Input: part model. Units: mm. Frame: model coordinates. A direction names the side the tool comes from. Coordinates: 2 decimals unless noted, no trailing zeros. Loops run counter-clockwise (first coordinate to the right, second up) from the corner with the lowest first, then second, coordinate; pieces in that order, holes last. Notation, with made-up numbers: M 32.25,-33.5 L 41.25,-33.5 A12 cw 41.25,-24.5 Z; hole C 8.5,6 d4. An arc over 180 degrees is marked long. Use a Markdown table: item, result. Add a question column.
1. Section D-D on x = -25.5. Output: boundary loops of the cut face in (y, z).
2. Set-up query: faces 1 (the cylindrical face through (-0.75, 5.7, 45.11)), 2 (the flat face through (-9.015, -2.652, 48.444)), 3 (the flat face through (-20.5, 1, 48)). Return all of +Z, -Z, +X, -X, +Y, -Y with unobstructed straight access to the full face (end or side cutting, diameter ignored); none if empty.
3. Pin query (flat end, axial travel): pin 1 (2 mm diameter, centred on x = -12.5, y = 0, fed in from -Z); pin 2 (3 mm diameter, centred on x = -35.5, z = 77.5, fed in from +Y); pin 3 (2 mm diameter, centred on x = -14.5, y = 0, fed in from +Z). Return the tip coordinate at first contact, or that it passes through.
4. Section C-C on z = 75. Output: boundary loops of the cut face in (x, y), then the cut area to 3 significant figures.
5. Draft query along Z for faces 4 (the flat face through (-10, 5.715, 48)), 5 (the flat face through (-10, -1, 47.1)), 6 (the flat face through (-36.45, -4.73, 75.52)). Return one class per face: +Z half, -Z half, draft (parallel to the pull), parting line (faces both ways), or undercut.
6. Section A-A on y = -3. Output: boundary loops of the cut face in (x, z), then the cut area to 3 significant figures.
7. Section B-B on x = -2.5. Output: boundary loops of the cut face in (y, z), then the cut area to 3 significant figures.
8. Line query: L1, parallel to Y at x = -17.5, z = 54; L2, parallel to Z at x = -15.5, y = 0; L3, parallel to Y at x = -6.5, z = 46.75. Output: solid intervals per line, ascending. Write a range as [from, to].
```python
from build123d import *

# Parameters (mm, degrees)
SKETCH045_R        = 5.75
SKETCH045_R_2      = 3.75
PAD013_DEPTH       = 2.25
PAD014_DEPTH       = 3.5
POCKET003048_DEPTH = 2.65
SKETCH048_R        = 3.75
SKETCH048_R_2      = 0.75
POCKET003049_DEPTH = 5
SKETCH050_R        = 1.25
PAD015_DEPTH       = 2


with BuildPart() as part:
    # Sketch045 → Pad013 (new body)
    with BuildSketch(Plane.XY):
        Circle(SKETCH045_R)
        Circle(SKETCH045_R_2, mode=Mode.SUBTRACT)
    extrude(amount=PAD013_DEPTH)

    # Sketch047 (on Face4 of Pad013) → Pad014 (join)
    with BuildSketch(Plane.XY.offset(2.25)):
        with BuildLine():
            Line((0, 5.714965), (-20.5, 5.714965))
            Line((-20.5, 5.714965), (-20.5, -5.714965))
            Line((0, -5.714965), (-20.5, -5.714965))
            ThreePointArc((0, -5.714965), (5.714965, 0), (0, 5.714965))
        make_face()
    extrude(amount=PAD014_DEPTH)

    # Sketch046 (on Face11 of Pad014) → Pocket003048 (cut)
    with BuildSketch(Plane.XY.offset(5.75)):
        with BuildLine():
            Line((-1.25, 3.535534), (-16.999999, 1.742953))
            ThreePointArc((-16.999999, 1.742953), (-18.232454, 1.232454), (-18.742953, 0))
            ThreePointArc((-18.742953, 0), (-18.232454, -1.232454), (-16.999999, -1.742953))
            Line((-1.25, -3.535534), (-16.999999, -1.742953))
            ThreePointArc((-1.25, -3.535534), (2.165064, -3.061862), (3.75, 0))
            ThreePointArc((3.75, 0), (2.165064, 3.061862), (-1.25, 3.535534))
        make_face()
    extrude(amount=-POCKET003048_DEPTH, mode=Mode.SUBTRACT)

    # Sketch048 (on Face16 of Pocket003048) → Pocket003049 (cut)
    with BuildSketch(Plane.XY.offset(3.1)):
        Circle(SKETCH048_R)
        with Locations((-14.5, 0)):
            Circle(SKETCH048_R_2)
        with Locations((-12.5, 0)):
            Circle(SKETCH048_R_2)
        with Locations((-10.5, 0)):
            Circle(SKETCH048_R_2)
        with Locations((-8.5, 0)):
            Circle(SKETCH048_R_2)
        with Locations((-6.5, 0)):
            Circle(SKETCH048_R_2)
    extrude(amount=-POCKET003049_DEPTH, mode=Mode.SUBTRACT)

    # Sketch050 (on Face2 of Pocket003049) → Pad015 (join)
    with BuildSketch(Plane.XZ.offset(5.714965)):
        with BuildLine():
            Line((-20.5, 2.25), (-43.255932, 25.005932))
            ThreePointArc((-43.255932, 33.234184), (-44.960058, 29.120058), (-43.255932, 25.005932))
            Line((-43.255932, 33.234184), (-38.30976, 38.180356))
            ThreePointArc((-29.532214, 38.180356), (-33.920987, 39.998245), (-38.30976, 38.180356))
            Line((-29.532214, 38.180356), (-3.425929, 12.074071))
            ThreePointArc((0, 3.803146), (-0.89037, 8.279338), (-3.425929, 12.074071))
            Line((0, 3.803146), (0, 2.25))
            Line((-20.5, 2.25), (0, 2.25))
        make_face()
        with Locations((-37.825367, 32.817886)):
            Circle(SKETCH050_R, mode=Mode.SUBTRACT)
        with Locations((-18.610336, 13.616402)):
            Circle(SKETCH050_R, mode=Mode.SUBTRACT)
        Polygon((-41.009785, 27.002425), (-31.760418, 36.165919), (-15.249238, 19.500009), (-24.498605, 10.336516), align=None, mode=Mode.SUBTRACT)
    extrude(amount=-PAD015_DEPTH)


with BuildPart() as part_1:
    # Body009 placement: moved
    add(part.part.moved(Location((0, 0, 44))))


solid = part_1.part
```
Answers below:
| question | item | result |
|---|---|---|
| 1 | outline | M -5.71,51.25 L -3.71,51.25 L -3.71,55.35 L -5.71,55.35 Z; M -5.71,73.85 L -3.71,73.85 L -3.71,78.15 L -5.71,78.15 Z |
| 2 | face 1 | -Z |
| 2 | face 2 | +Z |
| 2 | face 3 | +Z, -Z, -X, +Y |
| 3 | pin 1 | stops at z = 46.25 |
| 3 | pin 2 | stops at y = -3.71 |
| 3 | pin 3 | stops at z = 47.1 |
| 4 | outline | M -44.65,-5.71 L -36.97,-5.71 L -36.97,-3.71 L -44.65,-3.71 Z; M -26.64,-5.71 L -22.35,-5.71 L -22.35,-3.71 L -26.64,-3.71 Z |
| 4 | area | 23.9 mm² |
| 5 | face 4 | draft |
| 5 | face 5 | +Z half |
| 5 | face 6 | undercut |
| 6 | outline | M -20.5,46.25 L -4.91,46.25 L -4.91,44 L -2.25,44 L -2.25,47.1 L -5.96,47.1 L -5.96,49.75 L -20.5,49.75 Z; M 2.25,44 L 4.91,44 L 4.91,46.25 L 4.86,46.25 L 4.86,49.75 L 2.25,49.75 Z |
| 6 | area | 75.2 mm² |
| 7 | outline | M -5.71,46.25 L -5.18,46.25 L -5.18,44 L -2.8,44 L -2.8,47.1 L -3.39,47.1 L -3.39,49.75 L -3.71,49.75 L -3.71,55.03 L -5.71,55.03 Z; M 2.8,44 L 5.18,44 L 5.18,46.25 L 5.71,46.25 L 5.71,49.75 L 3.39,49.75 L 3.39,47.1 L 2.8,47.1 Z |
| 7 | area | 38.6 mm² |
| 8 | L1 | y = [-5.71, -3.71] |
| 8 | L2 | z = [46.25, 47.1] |
| 8 | L3 | y = [-5.71, -0.75], [0.75, 5.71] |
